Input: part model. Units: mm. Frame: model coordinates. A direction names the side the tool comes from. Round coordinates to 2 decimals unless told otherwise and drop trailing zeros. Loops run counter-clockwise (first coordinate to the right, second up) from the corner with the lowest first, then second, coordinate; pieces in that order, holes last. Notation, with made-up numbers: (1, 10.25) -> (59, 10.25) arc R5 cw to (59, 17.25) -> close; hole circle Ø10 at (86, 11.25). An arc over 180 degrees is marked (long way). Answer in a Markdown table with one row per item. Add a question column.
Q1. Section D-D, the plane z = -4.5. Output: boundary loops of the cut face in (x, y), and give its area (3 significant figures).
Q2. Section A-A, the plane z = 0. Output: boundary loops of the cut face in (x, y), and give its area (3 significant figures).
Q3. Ray query, L1, parallel to Y at x = 2, z = -14.5; L2, parallel to Y at x = -3, z = 5; L3, parallel to X at y = 55.1, z = 12.5. Return the intervals inside material, ascending. Write a range as from..to.
Q4. Mould query, pull axis Z, two halves, no side actions, for faces 1 (the face through (20, 0, 0)), 2 (the face through (19, -2, 3.5)), 3 (the face through (19, -4.5, 0)). Classes: pulls with the +Z half, pulls with the -Z half, needs draft (parallel to the pull), parting line crosses it, or undercut.
Q5. Pin query (flat end, axial travel): pin 1 (8 mm diameter, centred on x = -9.5, y = 5, fed in from +Z); pin 2 (3.5 mm diameter, centred on x = 19, y = -2.5, fed in from +Z); pin 3 (3.5 mm diameter, centred on x = -0.5, z = 12, fed in from +Y); pin 4 (14.5 mm diameter, centred on x = -1, z = 1.5, fed in from +Y). Return the tip coordinate at first contact, or that it passes through.
Q6. Section C-C, the plane y = 15. Output: boundary loops of the cut face in (x, z), and give its area (3 significant figures).
Q7. Section B-B, the plane x = 0. Output: boundary loops of the cut face in (y, z), and give its area (3 significant figures).
Q8. Reachability of faces 4 (the face through (8, 57, 0)), 5 (the face through (19, -3, -3)), 6 (the face through (19, -5, 0)), 7 (the face through (19, -2, -3.5)), 8 (the face through (10.74, -5.42, -2.38)) from +Z, -Z, +X, -X, +Y, -Y: full face, straight path, thin tool, end or side. Return the list, or none.
```python
from build123d import *

# Parameters (mm, degrees)
SKETCH_1_R          = 18.75
EXTRUDE_1_DEPTH     = 57
SKETCH_2_R          = 11
EXTRUDE_2_DEPTH     = 11
SKETCH_3_W          = 3
SKETCH_3_H          = 7
EXTRUDE_3_DEPTH     = 5
SKETCH_4_W          = 6
SKETCH_4_H          = 4
CUT_EXTRUDE_1_DEPTH = 3
SKETCH_5_R          = 6.5
EXTRUDE_4_DEPTH     = 4.5
SKETCH_6_R          = 1.6
CUT_EXTRUDE_2_DEPTH = 4
SKETCH_7_R          = 1.6
EXTRUDE_5_DEPTH     = 13.5


with BuildPart() as part:
    # 草图1 → 凸台-拉伸1 (new body)
    with BuildSketch(Plane(origin=(0, 0, 0), x_dir=(1, 0, 0), z_dir=(0, 1, 0))):
        with Locations(Location((0, 0, 0), (0, 0, 90))):
            Circle(SKETCH_1_R)
    extrude(amount=EXTRUDE_1_DEPTH)

    # 草图2 → 凸台-拉伸2 (add)
    with BuildSketch(Plane.XZ):
        with Locations(Location((0, 0, 0), (0, 0, 90))):
            Circle(SKETCH_2_R)
    extrude(amount=EXTRUDE_2_DEPTH)

    # 草图3 → 凸台-拉伸3 (add)
    with BuildSketch(Plane.XZ):
        with Locations((18.75, 0)):
            Rectangle(SKETCH_3_W, SKETCH_3_H)
    extrude(amount=EXTRUDE_3_DEPTH)

    # 草图4 → 切除-拉伸1 (cut)
    with BuildSketch(Plane(origin=(20.25, 0, 0), x_dir=(0, 0, -1), z_dir=(1, 0, 0))):
        with Locations((0, -2.5)):
            Rectangle(SKETCH_4_W, SKETCH_4_H)
    extrude(amount=-CUT_EXTRUDE_1_DEPTH, mode=Mode.SUBTRACT)

    # 草图5 → 凸台-拉伸4 (add)
    with BuildSketch(Plane(origin=(0, 57, 0), x_dir=(1, 0, 0), z_dir=(0, 1, 0))):
        with Locations(Location((0, 0, 0), (0, 0, 270))):
            Circle(SKETCH_5_R)
    extrude(amount=EXTRUDE_4_DEPTH)

    # 草图6 → 切除-拉伸2 (cut)
    with BuildSketch(Plane(origin=(0, 57, 0), x_dir=(1, 0, 0), z_dir=(0, 1, 0))):
        with Locations(Location((0, -12.5, 0), (0, 0, 270))):
            Circle(SKETCH_6_R)
        with Locations(Location((0, 12.5, 0), (0, 0, 270))):
            Circle(SKETCH_6_R)
    extrude(amount=-CUT_EXTRUDE_2_DEPTH, mode=Mode.SUBTRACT)

    # 草图7 → 凸台-拉伸5 (add)
    with BuildSketch(Plane(origin=(0, 61.5, 0), x_dir=(1, 0, 0), z_dir=(0, 1, 0))):
        with Locations(Location((0, 0, 0), (0, 0, 270))):
            Circle(SKETCH_7_R)
    extrude(amount=EXTRUDE_5_DEPTH)


solid = part.part
```
Answer block:
| question | item | result |
|---|---|---|
| 1 | outline | (-18.2, 0) -> (-10.04, 0) -> (-10.04, -11) -> (10.04, -11) -> (10.04, 0) -> (18.2, 0) -> (18.2, 57) -> (4.69, 57) -> (4.69, 61.5) -> (-4.69, 61.5) -> (-4.69, 57) -> (-18.2, 57) -> close |
| 1 | area | 2,340 mm^2 |
| 2 | outline | (-18.75, 0) -> (-11, 0) -> (-11, -11) -> (11, -11) -> (11, 0) -> (17.25, 0) -> (17.25, -0.5) -> (20.25, -0.5) -> (20.25, 0) -> (18.75, 0) -> (18.75, 57) -> (6.5, 57) -> (6.5, 61.5) -> (1.6, 61.5) -> (1.6, 75) -> (-1.6, 75) -> (-1.6, 61.5) -> (-6.5, 61.5) -> (-6.5, 57) -> (-18.75, 57) -> close; (17.25, -5) -> (20.25, -5) -> (20.25, -4.5) -> (17.25, -4.5) -> close |
| 2 | area | 2,480 mm^2 |
| 3 | L1 | 0..57 |
| 3 | L2 | -11..61.5 |
| 3 | L3 | -13.98..-1.6, 1.6..13.98 |
| 4 | face 1 | needs draft |
| 4 | face 2 | pulls with the +Z half |
| 4 | face 3 | undercut |
| 5 | pin 1 | z = 17.93 |
| 5 | pin 2 | z = 3.5 |
| 5 | pin 3 | y = 57 |
| 5 | pin 4 | y = 75 |
| 6 | outline | circle Ø37.5 at (0, 0) |
| 6 | area | 1,100 mm^2 |
| 7 | outline | (-11, -11) -> (0, -11) -> (0, -18.75) -> (57, -18.75) -> (57, -14.1) -> (53, -14.1) -> (53, -10.9) -> (57, -10.9) -> (57, -6.5) -> (61.5, -6.5) -> (61.5, -1.6) -> (75, -1.6) -> (75, 1.6) -> (61.5, 1.6) -> (61.5, 6.5) -> (57, 6.5) -> (57, 10.9) -> (53, 10.9) -> (53, 14.1) -> (57, 14.1) -> (57, 18.75) -> (0, 18.75) -> (0, 11) -> (-11, 11) -> close |
| 7 | area | 2,460 mm^2 |
| 8 | face 4 | +Y |
| 8 | face 5 | +X |
| 8 | face 6 | +Z, -Z, +X, -Y |
| 8 | face 7 | -Z, +X, -Y |
| 8 | face 8 | -Y |
